Could you check a few things on this model? Use its own coordinates, in mm. Face numbers are marked on the shaded views. A direction names the side the tool comes from. Coordinates: 2 decimals unless noted, no trailing zeros. Loops run counter-clockwise (first coordinate to the right, second up) from the corner with the lowest first, then second, coordinate; pieces in that order, holes last. Notation, with made-up numbers: (76.25, 64) - (85.25, 64) arc R19 ccw to (85.25, 83) - close; hole circle Ø1 at (2.25, 74.5). An arc over 180 degrees is marked (long way). One line per item, written item: value. Start each with the question number.
(1) If we section it at C-C on z = 8.5: Write out the boundary of the cut face in (x, y), then the cut area to 3 significant figures.
(2) If we mould it in two halves opening along Z, with no side actions, what happens to the marked faces 4, 5, 6 and 7? For each: pulls with the +Z half, pulls with the -Z half, needs draft (parallel to the pull), parting line crosses it, or undercut.
(3) If we section it at A-A on y = 9.5: Write out the boundary of the cut face in (x, z).
(4) If we section it at B-B on x = 19: Write out the boundary of the cut face in (y, z).
(5) On a 3-axis mill with a long thin cutter (end or side, diameter ignored), from which of +Z, -Z, +X, -X, +Y, -Y can I reach the whole of each face in a straight line? I mean the marked faces 1, 2 and 3. Say none if no direction works.
(6) I'm going to push flat-ended pins straight in: P1, Ø4, axis at x = 22.54, z = 36.36, coming from the +Y side; P2, Ø11, axis at y = 22, z = 37, coming from the -X side; P3, Ø5, axis at x = -1.96, z = -5.14, coming from the +Y side. Where does each tip first touch, or does it pass through?
(7) If we section it at D-D on x = 5.5: Write out the boundary of the cut face in (y, z), then the cut area to 3 significant figures.
(8) If I drill on line 1 along Z through (x, y) = (21, 30); line 2 along Z through (x, y) = (22.5, 3.5); line 3 along Y through (x, z) = (4.5, 27), over which ranges is the centre line in solid material (lowest first)? Write a range as from..to.
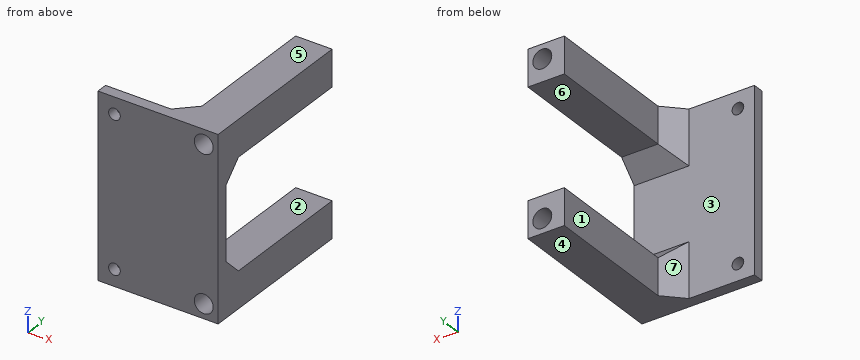
```python
from build123d import *

# Parameters (mm, degrees)
SKETCH1_R           = 1.6
BOSS_EXTRUDE1_DEPTH = 3
SKETCH2_W           = 10
SKETCH2_H           = 10
BOSS_EXTRUDE2_DEPTH = 42
CHAMFER1_SIZE       = 5
SKETCH3_R           = 2.6
CUT_EXTRUDE1_DEPTH  = 52


with BuildPart() as part:
    # Sketch1 → Boss-Extrude1 (new body)
    with BuildSketch(Plane(origin=(0, 0, 0), x_dir=(1, 0, 0), z_dir=(0, 1, 0))):
        Polygon((-6.512396694, 9.685950413), (1.487603306, 9.685950413), (26.487603306, 9.685950413), (26.487603306, -40.314049587), (1.487603306, -40.314049587), (-6.512396694, -40.314049587), align=None)
        with Locations(Location((-1.962396694, -35.764049587, 0), (0, 0, 270))):
            Circle(SKETCH1_R, mode=Mode.SUBTRACT)
        with Locations(Location((-1.962396694, 5.135950413, 0), (0, 0, 270))):
            Circle(SKETCH1_R, mode=Mode.SUBTRACT)
    extrude(amount=BOSS_EXTRUDE1_DEPTH)

    # Sketch2 → Boss-Extrude2 (add)
    with BuildSketch(Plane(origin=(0, 3, 0), x_dir=(1, 0, 0), z_dir=(0, 1, 0))):
        with Locations((21.487603306, -35.314049587)):
            Rectangle(SKETCH2_W, SKETCH2_H)
        with Locations((21.487603306, 4.685950413)):
            Rectangle(SKETCH2_W, SKETCH2_H)
    extrude(amount=BOSS_EXTRUDE2_DEPTH)

    # Chamfer1
    chamfer1_edges = [part.edges().sort_by_distance(p)[0] for p in [
        (21.487603306, 3, 30.314049587),
        (16.487603306, 3, 35.314049587),
        (16.487603306, 3, -4.685950413),
        (21.487603306, 3, 0.314049587),
    ]]
    chamfer(chamfer1_edges, length=CHAMFER1_SIZE)

    # Sketch3 → Cut-Extrude1 (cut)
    with BuildSketch(Plane(origin=(0, 45, 0), x_dir=(1, 0, 0), z_dir=(0, 1, 0))):
        with Locations(Location((22.537603306, -36.364049587, 0), (0, 0, 270))):
            Circle(SKETCH3_R)
        with Locations(Location((22.537603306, 5.735950413, 0), (0, 0, 270))):
            Circle(SKETCH3_R)
    extrude(amount=-CUT_EXTRUDE1_DEPTH, mode=Mode.SUBTRACT)


solid = part.part
```
Values:
1. outline: (-6.51, 0) - (26.49, 0) - (26.49, 3) - (-6.51, 3) - close
1. area: 99.0 mm2
2. face 4: pulls with the -Z half
2. face 5: pulls with the +Z half
2. face 6: undercut
2. face 7: needs draft
3. outline: (16.49, -9.69) - (26.49, -9.69) - (26.49, 0.31) - (16.49, 0.31) - close; (16.49, 30.31) - (26.49, 30.31) - (26.49, 40.31) - (16.49, 40.31) - close; hole circle Ø5.2 at (22.54, -5.74); hole circle Ø5.2 at (22.54, 36.36)
4. outline: (0, -9.69) - (45, -9.69) - (45, 0.31) - (8, 0.31) - (3, 5.31) - (3, 25.31) - (8, 30.31) - (45, 30.31) - (45, 40.31) - (0, 40.31) - close
5. face 1: +Z, -Z, -X, +Y
5. face 2: +X, -X, +Y
5. face 3: -X, +Y
6. P1: passes through
6. P2: stops at x = 16.49
6. P3: stops at y = 3
7. outline: (0, -9.69) - (3, -9.69) - (3, 40.31) - (0, 40.31) - close
7. area: 150 mm2
8. line 1: z = -9.69..-7.83, -3.64..0.31, 30.31..34.27, 38.46..40.31
8. line 2: z = -9.69..-8.34, -3.14..4.81, 25.81..33.76, 38.96..40.31
8. line 3: y = 0..3
